Print and shaded views of the part. All mm, measured from the part's lowest x, y and z. Coordinates: 2 decimals unless noted, no trailing zeros. Order: outer loops, then holes, each group sorted by start corner. A loop starts at its lowest first (then second) coordinate and runs counter-clockwise, first axis right, second up. Notation, with made-up numbers: M 25.25,72 L 84.25,72 A25 ccw 84.25,87 Z; hole C 60.25,26 d11. An arc over 180 degrees is marked long. Return JSON: item names as keys, results as strings.
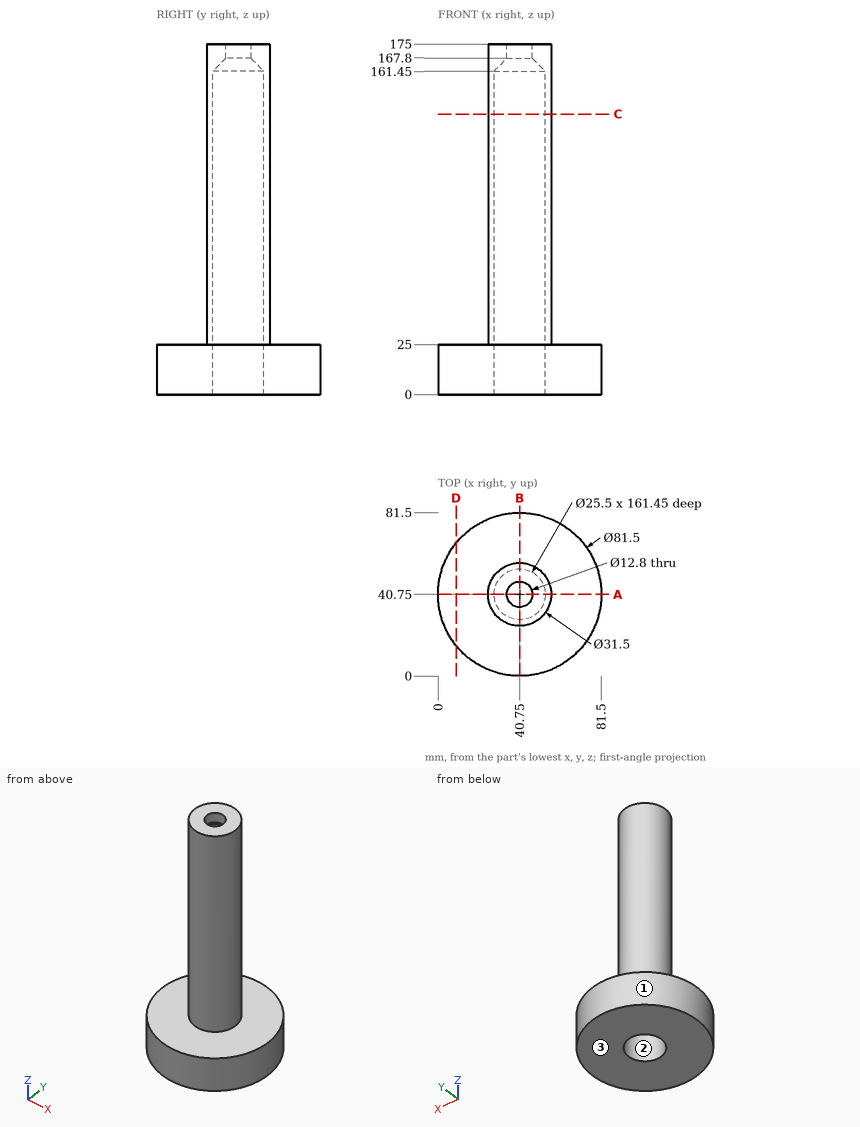
Item 1: Saw through at A-A (y = 40.75). Write the cut outline in (x, z).
Check result:
{"outline": "M 0,0 L 28,0 L 28,161.45 L 34.35,167.8 L 34.35,175 L 25,175 L 25,25 L 0,25 Z; M 47.15,167.8 L 53.5,161.45 L 53.5,0 L 81.5,0 L 81.5,25 L 56.5,25 L 56.5,175 L 47.15,175 Z"}
Item 2: Pull direction X, two halves, no side cores. Call the marked faces 1, 2 and 3: +X half, -X half, draft (parallel to the pull), parting line (faces both ways), or undercut.
Check result:
{"face 1": "parting line", "face 2": "undercut", "face 3": "draft"}
Item 3: Drop flat-ended pins along their axis: pin 1 Ø8 at (y, z) = (39.5, 123.5) entering from +X; pin 2 Ø10 at (x, z) = (28.5, 29) entering from -Y; pin 3 Ø1 at (y, z) = (33.5, 154.5) entering from +X. Give the stop position or say it passes through.
Check result:
{"pin 1": "stops at x = 56.5", "pin 2": "stops at y = 1.06", "pin 3": "stops at x = 54.98"}
Item 4: Saw through at D-D (x = 9). Write the cut outline in (y, z), and give its area (3 significant figures).
Check result:
{"outline": "M 15.21,0 L 66.29,0 L 66.29,25 L 15.21,25 Z", "area": "1,280 mm2"}
Item 5: Wall check: line 1 (Z direction, x = 38.5, y = 68); line 2 (X direction, y = 45, z = 166.5); line 3 (Y direction, x = 31, z = 67.5). Give the ranges that are in metal, low to high.
Check result:
{"line 1": "z = 0 to 25", "line 2": "x = 25.58 to 34.33, 47.17 to 55.92", "line 3": "y = 28.38 to 32.53, 48.97 to 53.12"}
Item 6: Saw through at C-C (z = 140). Write the cut outline in (x, y), and give its area (3 significant figures).
Check result:
{"outline": "C 40.75,40.75 d31.5; hole C 40.75,40.75 d25.5", "area": "269 mm2"}
